```python
from build123d import *

# Parameters (mm, degrees)
F1_DEPTH = 63.5
F2_DEPTH = 25.4
F3_DEPTH = 8.255
F5_R     = 6.35


with BuildPart() as f1:
    # F0 (on Front) → F1 (new body, symmetric)
    with BuildSketch(Plane.XZ):
        Polygon((-41.275, -9.525), (41.275, -9.525), (41.275, 9.525), (22.225, 9.525), (-41.275, 9.525), align=None)
    extrude(amount=F1_DEPTH, both=True)

    # F0 (on Front) → F2 (join, symmetric)
    with BuildSketch(Plane.XZ):
        with BuildLine():
            Line((22.225, 9.525), (41.275, 9.525))
            Line((41.275, 9.525), (41.275, 27.0002))
            ThreePointArc((41.275, 27.0002), (45.92468, 38.22552), (57.15, 42.8752))
            Line((57.15, 42.8752), (60.325, 42.8752))
            Line((60.325, 42.8752), (60.325, 61.9252))
            Line((60.325, 61.9252), (57.15, 61.9252))
            ThreePointArc((57.15, 61.9252), (32.454296, 51.695904), (22.225, 27.0002))
            Line((22.225, 27.0002), (22.225, 9.525))
        make_face()
        Polygon((85.748255, 61.9252), (60.325, 61.9252), (60.325, 42.8752), (60.325, 34.925), (85.748255, 34.925), align=None)
    extrude(amount=F2_DEPTH, both=True)

    # F0 (on Front) → F3 (join, symmetric)
    with BuildSketch(Plane.XZ):
        with BuildLine():
            add(Edge.make_bspline(
                [(-41.275, 9.525), (-33.85127, 45.177106), (16.302885, 62.071145), (57.15, 61.9252)],
                knots=[0, 0, 0, 0, 111.504536, 111.504536, 111.504536, 111.504536], degree=3))
            Line((-41.275, 9.525), (22.225, 9.525))
            Line((22.225, 9.525), (22.225, 27.0002))
            ThreePointArc((22.225, 27.0002), (32.454296, 51.695904), (57.15, 61.9252))
        make_face()
    extrude(amount=F3_DEPTH, both=True)

    # F0 (on Front) → F4 (revolve)
    with BuildSketch(Plane.XZ):
        Polygon((85.748255, 66.675), (85.748255, 61.9252), (85.748255, 34.925), (111.125, 34.925), (111.125, 66.675), align=None)
    revolve(axis=Axis((85.748255, 0, 50.8), (0, 0, -1)))

    # F5
    f5_edges = [f1.edges().sort_by_distance(p)[0] for p in [
        (-41.275, -63.5, 0),
        (41.275, -63.5, 0),
        (41.275, 63.5, 0),
        (-41.275, 63.5, 0),
        (-1.167948, 8.255, 50.677931),
        (-1.167948, -8.255, 50.677931),
    ]]
    fillet(f5_edges, radius=F5_R)


solid = f1.part
```
The model under review builds one solid part; all positions refer to its coordinate system, in mm. A direction names the side the tool comes from. Round coordinates to 2 decimals unless told otherwise and drop trailing zeros. Order: outer loops, then holes, each group sorted by start corner. A loop starts at its lowest first (then second) coordinate and runs counter-clockwise, first axis right, second up.
Item 1: Add section C-C, the plane y = -37. State the section outline as (x, z) points (3 decimals).
Working result:
outline: (-41.275, -9.525) - (41.275, -9.525) - (41.275, 9.525) - (-41.275, 9.525) - close
Item 2: Draft analysis for pull direction X (two halves, no side actions). For faces 1 (the cylindrical face through (45.8, -0.4, 38.1)), 2 (the flat face through (22.225, -17, 18)), 3 (the flat face through (46, -25.4, 42)), state which applies: released by +X, released by -X, zero draft, split by the parting line, or undercut.
Working result:
face 1: undercut
face 2: released by -X
face 3: zero draft
Item 3: Machinability: for faces 4 (the cylindrical face through (32.73, -16.43, 51.97)), 5 (the cylindrical face through (109.953, -7.622, 51.022)), 6 (the flat face through (22.225, 17, 18)), which of the approach directions +Z, -Z, +X, -X, +Y, -Y give a long, thin tool a straight path to every point of the face, cutting with its end or side? Answer none if there is none.
Working result:
face 4: +Z, -X, -Y
face 5: +Z
face 6: +Z, -X, +Y
Item 4: To check wall thickness, follow probe 1 along Y at (x, z) = (74, 54.5); probe 2 along X at (y, z) = (-8.5, 7.5) (3 decimals); probe 3 along Z at (x, y) = (95.5, -1.5) (3 decimals). State the ranges of each line that lie inside material, in increasing order.
Working result:
probe 1: y = -25.4 to 25.4
probe 2: x = -41.275 to 41.275
probe 3: z = 34.925 to 66.675
Item 5: For pin 1 (6.5 mm diameter, centred on y = 6.5, z = 38.5, fed in from -X); pin 2 (8 mm diameter, centred on x = 94, z = 33.5, fed in from +Y); pin 3 (3.5 mm diameter, centred on x = 59.5, y = -2.5, fed in from -Z) (3 decimals), all flat-tipped, find the tip position at first contact; note any pin that passes through.
Working result:
pin 1: stops at x = -24.39
pin 2: stops at y = 24.97
pin 3: stops at z = 34.925
Item 6: Add section B-B, the plane x = 79.5. State the section outline as (y, z) points (1 decimal).
Working result:
outline: (-25.4, 34.9) - (25.4, 34.9) - (25.4, 61.9) - (24.6, 61.9) - (24.6, 66.7) - (-24.6, 66.7) - (-24.6, 61.9) - (-25.4, 61.9) - close
